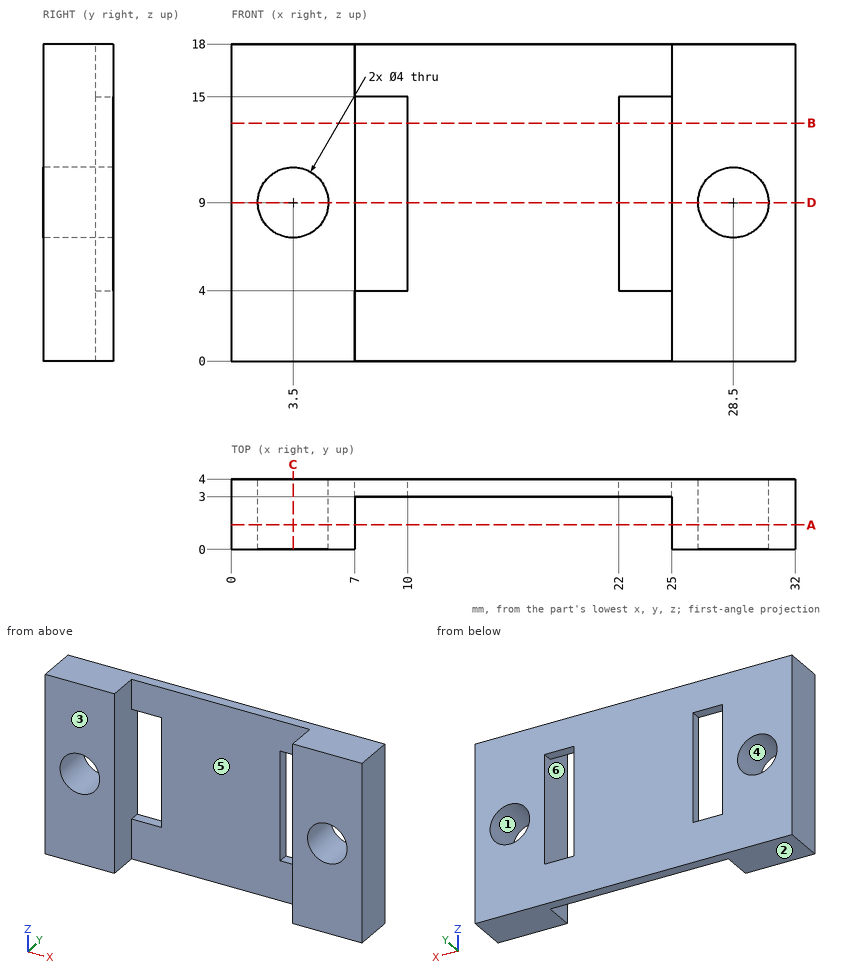
Verification items for this drawing (mm, ordinates from the low corner). A direction names the side the tool comes from. Give positions to 0.01 mm unless a question says otherwise; leave off trailing zeros. Loops run counter-clockwise (first coordinate to the right, second up) from the corner with the lowest first, then second, coordinate; pieces in that order, holes last. Notation, with made-up numbers: M 51.25,37.25 L 75.25,37.25 A11 ccw 75.25,44.25 Z; hole C -10,-28.75 d7. An arc over 180 degrees is marked long. Return JSON: item names as keys, results as strings. Group by question number.
1. Go/stop test with a flat-tipped pin: pin 1 (9 mm diameter, centred on x = 19, z = 9, fed in from -Y). Record where the tip stops, or that it passes through.
2. Cross-section at B-B on z = 13.5. Record the boundary of the cut face in (x, y), plus the area to 3 significant figures.
3. Cross-section at A-A on y = 1.4. Record the boundary of the cut face in (x, z), plus the area to 3 significant figures.
4. Cross-section at C-C on x = 3.5. Record the boundary of the cut face in (y, z).
5. Tool access check on the marked faces 4, 5 and 6. Record the directions out of +Z, -Z, +X, -X, +Y, -Y that give a thin tool (end or side, any length) a straight path to the whole face; none if there is none.
6. Cross-section at D-D on z = 9. Record the boundary of the cut face in (x, y).
7. Mould release check, pull along Z, two halves, no side actions. Record for the marked faces 1, 2 and 3: released by +Z, released by -Z, zero draft, split by the parting line, or undercut.
8. Thickness scan on L1, parallel to X at y = 2.2, z = 9; L2, parallel to Z at x = 23, y = 3.8; L3, parallel to Z at x = 28.5, y = 2.65. Record the ranges inside material, lowest first.
Return value:
{
 "1": {"pin 1": "y = 3"},
 "2": {"outline": "M 0,0 L 7,0 L 7,4 L 0,4 Z; M 10,3 L 22,3 L 22,4 L 10,4 Z; M 25,0 L 32,0 L 32,4 L 25,4 Z", "area": "68.0 mm^2"},
 "3": {"outline": "M 0,0 L 7,0 L 7,18 L 0,18 Z; M 25,0 L 32,0 L 32,18 L 25,18 Z; hole C 3.5,9 d4; hole C 28.5,9 d4", "area": "227 mm^2"},
 "4": {"outline": "M 0,0 L 4,0 L 4,7 L 0,7 Z; M 0,11 L 4,11 L 4,18 L 0,18 Z"},
 "5": {"face 4": "+Y, -Y", "face 5": "+Z, -Z, -Y", "face 6": "-Y"},
 "6": {"outline": "M 0,0 L 1.5,0 L 1.5,4 L 0,4 Z; M 5.5,0 L 7,0 L 7,4 L 5.5,4 Z; M 10,3 L 22,3 L 22,4 L 10,4 Z; M 25,0 L 26.5,0 L 26.5,4 L 25,4 Z; M 30.5,0 L 32,0 L 32,4 L 30.5,4 Z"},
 "7": {"face 1": "undercut", "face 2": "released by -Z", "face 3": "zero draft"},
 "8": {"L1": "0 to 1.5, 5.5 to 7, 25 to 26.5, 30.5 to 32", "L2": "0 to 4, 15 to 18", "L3": "0 to 7, 11 to 18"}
}
